Input: dimensioned drawing with shaded views. Units: mm. Origin: part minimum x, y, z. A direction names the side the tool comes from. Coordinates: 2 decimals unless noted, no trailing zeros. Loops run counter-clockwise (first coordinate to the right, second up) from the corner with the lowest first, then second, coordinate; pieces in that order, holes last.
Item 1: Section query A-A, the plane z = 13. Return the cut outline in (x, y), then the cut area to 3 significant figures.
Item 2: Line query: probe 1 along X at (y, z) = (1.2, 13); probe 2 along Z at (x, y) = (40, 1.75); probe 3 along X at (y, z) = (5.7, 18.5). Output: solid intervals per line, ascending.
Item 3: Section query B-B, the plane y = 1.3. Return the cut outline in (x, z), then the cut area to 3 significant figures.
Item 4: Pin query (flat end, axial travel): pin 1 Ø1.6 at (y, z) = (5.5, 8) entering from -X; pin 2 Ø4.5 at (x, z) = (10, 13) entering from +Y; pin 3 Ø8 at (x, z) = (27, 15.5) entering from +Y; pin 4 Ø1 at (y, z) = (5, 17) entering from +X. Return the tip coordinate at first contact, or that it passes through.
Item 5: Section query C-C, the plane x = 10. Return the cut outline in (y, z).
Item 6: Reachability of the marked faces 4, 5 and 6 from +Z, -Z, +X, -X, +Y, -Y: full face, straight path, thin tool, end or side. Return the list, or none.
Item 7: Section query D-D, the plane x = 18. Return the cut outline in (y, z), then the cut area to 3 significant figures.
Item 8: Pull-direction query (X, two-part tool) for the marked faces 1, 2 and 3; classes: +X half, -X half, draft (parallel to the pull), parting line (faces both ways), or undercut.
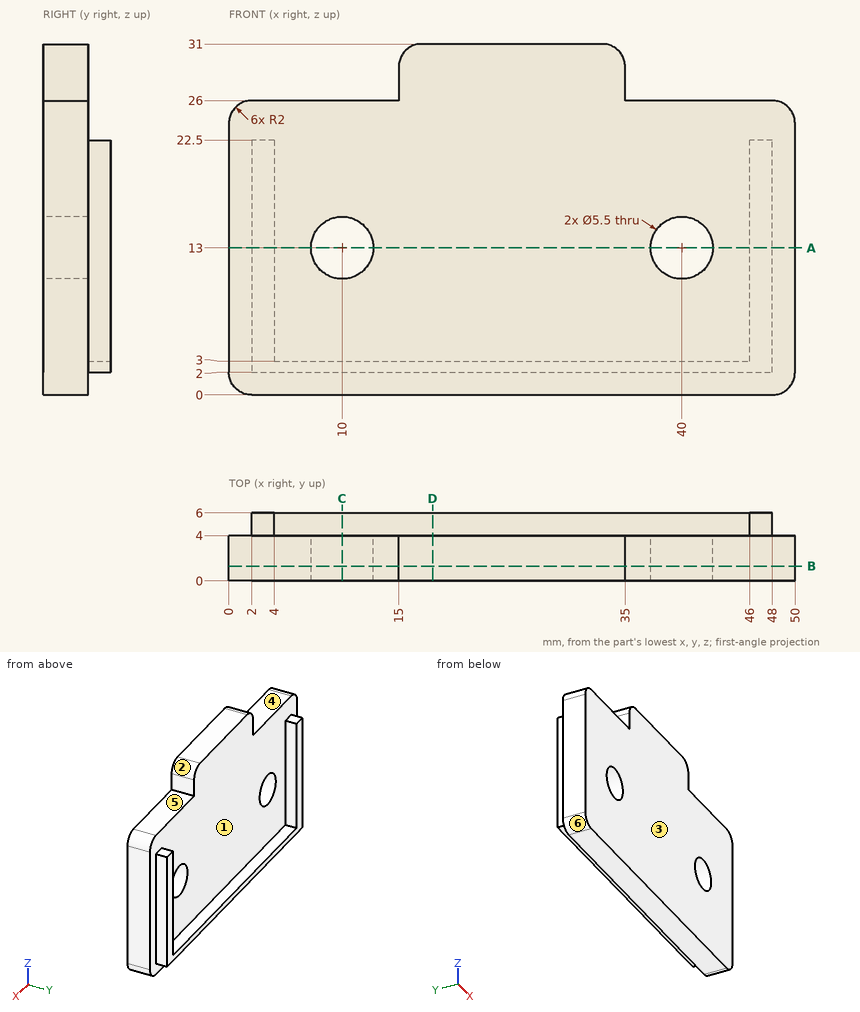
Verdict:
1. outline: (0, 0) - (7.25, 0) - (7.25, 4) - (4, 4) - (4, 6) - (2, 6) - (2, 4) - (0, 4) - close; (12.75, 0) - (37.25, 0) - (37.25, 4) - (12.75, 4) - close; (42.75, 0) - (50, 0) - (50, 4) - (48, 4) - (48, 6) - (46, 6) - (46, 4) - (42.75, 4) - close
1. area: 164 mm2
2. probe 1: x = 0 to 7.25, 12.75 to 37.25, 42.75 to 50
2. probe 2: z = 0 to 10.25, 15.75 to 26
2. probe 3: x = 2 to 4, 46 to 48
3. outline: (0, 2) arc R2 ccw to (2, 0) - (48, 0) arc R2 ccw to (50, 2) - (50, 24) arc R2 ccw to (48, 26) - (35, 26) - (35, 29) arc R2 ccw to (33, 31) - (17, 31) arc R2 ccw to (15, 29) - (15, 26) - (2, 26) arc R2 ccw to (0, 24) - close; hole circle Ø5.5 at (10, 13); hole circle Ø5.5 at (40, 13)
3. area: 1,350 mm2
4. pin 1: stops at x = 2
4. pin 2: passes through
4. pin 3: stops at y = 4
4. pin 4: stops at x = 48
5. outline: (0, 0) - (4, 0) - (4, 2) - (6, 2) - (6, 3) - (4, 3) - (4, 10.25) - (0, 10.25) - close; (0, 15.75) - (4, 15.75) - (4, 26) - (0, 26) - close
6. face 4: +Z, -X, +Y, -Y
6. face 5: +Z, +X, +Y, -Y
6. face 6: -Z, -X, +Y, -Y
7. outline: (0, 0) - (4, 0) - (4, 2) - (6, 2) - (6, 3) - (4, 3) - (4, 31) - (0, 31) - close
7. area: 126 mm2
8. face 1: undercut
8. face 2: +X half
8. face 3: draft
